Read the model definition and answer for the solid it produces. Units are mm, in the model's axes. Give positions to 0.01 mm unless a question says otherwise; leave off trailing zeros. Write each loop counter-clockwise with the first axis right and the second up, starting at its lowest first coordinate (ties: lowest second). Pieces come first, ordered by that corner, then holes. Notation, with made-up numbers: (58, 36) -> (73, 36) arc R27 cw to (73, 71) -> close; hole circle Ø9 at (-23.75, 13). An arc over 180 degrees is marked (long way). Use a Markdown table: item, result.
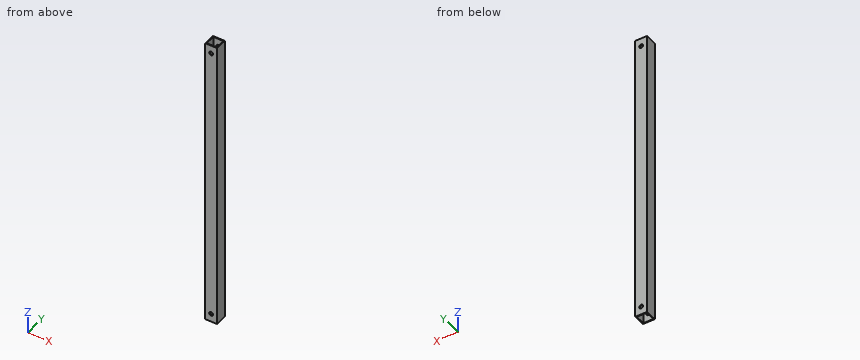
from build123d import *

# Parameters (mm, degrees)
SKIZZE1_W                       = 20
SKIZZE1_H                       = 20
SKIZZE1_W_2                     = 17
SKIZZE1_H_2                     = 17
AUFSATZ_LINEAR_AUSTRAGEN1_DEPTH = 250
SKIZZE2_R                       = 3.25
SCHNITT_LINEAR_AUSTRAGEN1_DEPTH = 15


with BuildPart() as part:
    # Skizze1 → Aufsatz-Linear austragen1 (new, symmetric)
    with BuildSketch(Plane.XY):
        Rectangle(SKIZZE1_W, SKIZZE1_H)
        Rectangle(SKIZZE1_W_2, SKIZZE1_H_2, mode=Mode.SUBTRACT)
    extrude(amount=AUFSATZ_LINEAR_AUSTRAGEN1_DEPTH, both=True)

    # Skizze2 → Schnitt-Linear austragen1 (cut, symmetric)
    with BuildSketch(Plane(origin=(0, 0, 0), x_dir=(1, 0, 0), z_dir=(0, 1, 0))):
        with Locations((0, -236)):
            Circle(SKIZZE2_R)
        with Locations((0, 236)):
            Circle(SKIZZE2_R)
    extrude(amount=SCHNITT_LINEAR_AUSTRAGEN1_DEPTH, both=True, mode=Mode.SUBTRACT)


solid = part.part
Item 1: A cutting plane is placed at A-A (y = -3.25). Give the vertices of the cut face in (x, z).
Return value:
| item | result |
|---|---|
| outline | (-10, -250) -> (-8.5, -250) -> (-8.5, 250) -> (-10, 250) -> close; (8.5, -250) -> (10, -250) -> (10, 250) -> (8.5, 250) -> close |
Item 2: A cutting plane is placed at B-B (z = -199.5). Give the vertices of the cut face in (x, y), then the cut area to 3 significant figures.
Return value:
| item | result |
|---|---|
| outline | (-10, -10) -> (10, -10) -> (10, 10) -> (-10, 10) -> close; hole (-8.5, -8.5) -> (8.5, -8.5) -> (8.5, 8.5) -> (-8.5, 8.5) -> close |
| area | 111 mm^2 |
Item 3: A cutting plane is placed at C-C (x = 0). Give the vertices of the cut face in (y, z).
Return value:
| item | result |
|---|---|
| outline | (-10, -250) -> (-8.5, -250) -> (-8.5, -239.25) -> (-10, -239.25) -> close; (-10, -232.75) -> (-8.5, -232.75) -> (-8.5, 232.75) -> (-10, 232.75) -> close; (-10, 239.25) -> (-8.5, 239.25) -> (-8.5, 250) -> (-10, 250) -> close; (8.5, -250) -> (10, -250) -> (10, -239.25) -> (8.5, -239.25) -> close; (8.5, -232.75) -> (10, -232.75) -> (10, 232.75) -> (8.5, 232.75) -> close; (8.5, 239.25) -> (10, 239.25) -> (10, 250) -> (8.5, 250) -> close |
Item 4: Straight lines are drawn through the part: line 1 along Z through (x, y) = (0, 9.15); line 2 along Y through (x, z) = (4.25, 152.5). For each, find the intervals that lie inside material, in ascending order. Write a range as [from, to].
Return value:
| item | result |
|---|---|
| line 1 | [-250, -239.25], [-232.75, 232.75], [239.25, 250] |
| line 2 | [-10, -8.5], [8.5, 10] |
